```python
from build123d import *

# Parameters (mm, degrees)
BOSS_EXTRUDE2_DEPTH = 5
SKETCH8_R           = 50
CUT_EXTRUDE6_DEPTH  = 20
SKETCH9_OUTSIDE_W   = 10.609
SKETCH9_OUTSIDE_H   = 17.306
SKETCH9_OUTSIDE_R   = 50
CUT_EXTRUDE7_DEPTH  = 20
SKETCH11_W          = 2
SKETCH11_H          = 8
SKETCH11_W_2        = 7
BOSS_EXTRUDE4_DEPTH = 2
CUT_EXTRUDE8_DEPTH  = 18
SKETCH13_R          = 0.3
CUT_EXTRUDE10_DEPTH = 20.940160481
SKETCH14_R          = 0.3
CUT_EXTRUDE11_DEPTH = 20
FILLET1_R           = 0.57
SKETCH15_R          = 16.5
CUT_EXTRUDE12_DEPTH = 20.940160481
SKETCH16_W          = 3.5
SKETCH16_H          = 4.171301815
SKETCH16_H_2        = 4.584730653
CUT_EXTRUDE14_DEPTH = 3.5


# Read off the part's stored shape, not the designer's step: Cut-Extrude8
with BuildPart() as part:
    # Sketch1 → Boss-Extrude2 (new body)
    with BuildSketch(Plane.XY):
        Polygon((0, 0), (0, 8), (2, 8), (2, 5), (5.5, 6), (5.5, 8), (12.5, 8), (12.5, 6), (16, 5), (16, 8), (18, 8), (18, 0), (16, 0), (16, -3), (12.5, -2), (12.5, 0), (5.5, 0), (5.5, -2), (2, -3), (2, 0), align=None)
    extrude(amount=BOSS_EXTRUDE2_DEPTH)

    # Sketch8 → Cut-Extrude6 (cut)
    with BuildSketch(Plane(origin=(0, 0, 0), x_dir=(0, 0, -1), z_dir=(1, 0, 0))):
        with Locations((49, 2.5)):
            Circle(SKETCH8_R)
    extrude(amount=CUT_EXTRUDE6_DEPTH, mode=Mode.SUBTRACT)

    # Sketch9 outside → Cut-Extrude7 (cut)
    with BuildSketch(Plane(origin=(0, 0, 0), x_dir=(0, 0, -1), z_dir=(1, 0, 0))):
        with Locations((-2.8485, 2.5)):
            Rectangle(SKETCH9_OUTSIDE_W, SKETCH9_OUTSIDE_H)
        with Locations((47.1, 2.5)):
            Circle(SKETCH9_OUTSIDE_R, mode=Mode.SUBTRACT)
    extrude(amount=CUT_EXTRUDE7_DEPTH, mode=Mode.SUBTRACT)

    # Sketch11 → Boss-Extrude4 (add)
    with BuildSketch(Plane.XY.offset(4)):
        with Locations((1, 4)):
            Rectangle(SKETCH11_W, SKETCH11_H)
        with Locations((9, 4)):
            Rectangle(SKETCH11_W_2, SKETCH11_H)
        with Locations((17, 4)):
            Rectangle(SKETCH11_W, SKETCH11_H)
    extrude(amount=-BOSS_EXTRUDE4_DEPTH)

    # Cut-Extrude8 outline → Cut-Extrude8 (cut)
    with BuildSketch(Plane(origin=(0, 0, 0), x_dir=(0, 0, -1), z_dir=(1, 0, 0))):
        with BuildLine():
            Line((-4, 0), (-3.037460889, 0))
            ThreePointArc((-3.037460889, 0), (-3.07734981, 4.004827558), (-2.796579359, 8))
            Line((-2.796579359, 8), (-4, 8))
            Line((-4, 8), (-4, 0))
        make_face()
    extrude(amount=CUT_EXTRUDE8_DEPTH, mode=Mode.SUBTRACT)

    # Sketch13 → Cut-Extrude10 (cut, through all)
    with BuildSketch(Plane(origin=(0, 0, 0), x_dir=(0, 0, -1), z_dir=(1, 0, 0))):
        with Locations(Location((-1.799307082, 7.02, 0), (0, 0, 270))):
            Circle(SKETCH13_R)
    extrude(amount=CUT_EXTRUDE10_DEPTH, mode=Mode.SUBTRACT)

    # Sketch14 → Cut-Extrude11 (cut)
    with BuildSketch(Plane(origin=(0, 0, 0), x_dir=(0, 0, -1), z_dir=(1, 0, 0))):
        with Locations(Location((-1.865607241, -1.2, 0), (0, 0, 270))):
            Circle(SKETCH14_R)
    extrude(amount=CUT_EXTRUDE11_DEPTH, mode=Mode.SUBTRACT)

    # Fillet1
    # the kernel refuses this fillet: 0.57 mm, written as the material it takes off along each edge
    with BuildSketch(Plane(origin=(16, 0, 3.037460889), x_dir=(0, 0, -1), z_dir=(1, 0, 0))) as fillet1_piece_1:
        with BuildLine():
            CenterArc((0.545153795, 0.57), FILLET1_R, 182.237689069, 87.762310931)
            ThreePointArc((-0.02441155, 0.547744285), (-0.012956585, 0.273838681), (0, 0))
            Line((0, 0), (0.545153795, 0))
        make_face()
    extrude(amount=3.370719987, mode=Mode.SUBTRACT)
    with BuildSketch(Plane(origin=(14.71001217, 8, 2.796579359), x_dir=(0, 0, -1), z_dir=(1, 0, 0)), Plane(origin=(-1.28998783, 8, 2.796579359), x_dir=(0, 0, -1), z_dir=(1, 0, 0))) as fillet1_piece_2:
        with BuildLine():
            CenterArc((0.513045529, -0.57), FILLET1_R, 90, 84.275973917)
            ThreePointArc((-0.054112356, -0.513149909), (-0.02771814, -0.25650515), (0, 0))
            Line((0, 0), (0.513045529, 0))
        make_face()
    extrude(amount=4.57997566, mode=Mode.SUBTRACT)
    with BuildSketch(Plane(origin=(5.5, 0, 3.037460889), x_dir=(0, 0, -1), z_dir=(1, 0, 0))) as fillet1_piece_3:
        with BuildLine():
            CenterArc((0.545153795, 0.57), FILLET1_R, 182.237689069, 87.762310931)
            ThreePointArc((-0.02441155, 0.547744285), (-0.012956585, 0.273838681), (0, 0))
            Line((0, 0), (0.545153795, 0))
        make_face()
    extrude(amount=7, mode=Mode.SUBTRACT)
    with BuildSketch(Plane(origin=(4.21001217, 8, 2.796579359), x_dir=(0, 0, -1), z_dir=(1, 0, 0))) as fillet1_piece_4:
        with BuildLine():
            CenterArc((0.513045529, -0.57), FILLET1_R, 90, 84.275973917)
            ThreePointArc((-0.054112356, -0.513149909), (-0.02771814, -0.25650515), (0, 0))
            Line((0, 0), (0.513045529, 0))
        make_face()
    extrude(amount=9.57997566, mode=Mode.SUBTRACT)
    with BuildSketch(Plane(origin=(-1.370719987, 0, 3.037460889), x_dir=(0, 0.9990083494743675, 0.044523226303807895), z_dir=(1, 0, 0))) as fillet1_piece_5:
        with BuildLine():
            CenterArc((0.545162753, -0.569991432), FILLET1_R, 89.685852545, 87.762310931)
            Line((-0.024272006, -0.544613193), (0, 0))
            ThreePointArc((0, 0), (0.274143997, 0.000751555), (0.548287995, 0))
        make_face()
    extrude(amount=3.370719987, mode=Mode.SUBTRACT)
    with BuildSketch(Plane(origin=(2, 0, 0.937460889), x_dir=(0, 0.9990278617443559, 0.04408323330360469), z_dir=(-1, 0, 0)), Plane(origin=(19.489241357, 0, 0.937460889), x_dir=(0, 0.9990278617443559, 0.04408323330360409), z_dir=(-1, 0, 0))) as fillet1_piece_6:
        with BuildLine():
            CenterArc((0.595706111, -0.569990001), FILLET1_R, 90.339381978, 92.187220026)
            Line((0.02626023, -0.595117444), (0, 0))
            ThreePointArc((0, 0), (0.296164915, -0.000877144), (0.592329831, 0))
        make_face()
    extrude(amount=3.489241357, mode=Mode.SUBTRACT)
    with BuildSketch(Plane(origin=(3.581343655, 8, 0.696579359), x_dir=(0, 0, 1), z_dir=(-1, 0, 0))) as fillet1_piece_7:
        with BuildLine():
            CenterArc((0.632537462, -0.57), FILLET1_R, 90, 95.594572842)
            ThreePointArc((0.065252578, -0.625568519), (0.033609947, -0.312681655), (0, 0))
            Line((0, 0), (0.632537462, 0))
        make_face()
    extrude(amount=5.16268731, mode=Mode.SUBTRACT)
    with BuildSketch(Plane(origin=(14.081343655, 8, 0.696579359), x_dir=(0, -0.9946037861150897, 0.1037463669027923), z_dir=(-1, 0, 0))) as fillet1_piece_8:
        with BuildLine():
            CenterArc((0.632547622, 0.569988725), FILLET1_R, 174.045055794, 95.594572842)
            Line((0.065623464, 0.629124155), (0, 0))
            ThreePointArc((0, 0), (0.314481268, 0.000988994), (0.628962535, 0))
        make_face()
    extrude(amount=10.16268731, mode=Mode.SUBTRACT)
    with BuildSketch(Plane(origin=(19.581343655, 8, 0.696579359), x_dir=(0, -0.9946037861150897, 0.1037463669027923), z_dir=(-1, 0, 0))) as fillet1_piece_9:
        with BuildLine():
            CenterArc((0.632547622, 0.569988725), FILLET1_R, 174.045055794, 95.594572842)
            Line((0.065623464, 0.629124155), (0, 0))
            ThreePointArc((0, 0), (0.314481268, 0.000988994), (0.628962535, 0))
        make_face()
    extrude(amount=5.16268731, mode=Mode.SUBTRACT)
    with BuildSketch(Plane(origin=(12.5, 0, 0.937460889), x_dir=(0, 0.9990278617443559, 0.04408323330360469), z_dir=(-1, 0, 0))) as fillet1_piece_10:
        with BuildLine():
            CenterArc((0.595706111, -0.569990001), FILLET1_R, 90.339381978, 92.187220026)
            Line((0.02626023, -0.595117444), (0, 0))
            ThreePointArc((0, 0), (0.296164915, -0.000877144), (0.592329831, 0))
        make_face()
    extrude(amount=7, mode=Mode.SUBTRACT)

    # Sketch15 → Cut-Extrude12 (cut, through all)
    with BuildSketch(Plane.XY):
        with Locations((9, -11.34889303)):
            Circle(SKETCH15_R)
    extrude(amount=CUT_EXTRUDE12_DEPTH, mode=Mode.SUBTRACT)

    # Sketch16 → Cut-Extrude14 (cut)
    with BuildSketch(Plane.XY.offset(5.6)):
        with Locations((3.75, 4.184345942)):
            Rectangle(SKETCH16_W, SKETCH16_H)
        with Locations((14.25, 4.391060361)):
            Rectangle(SKETCH16_W, SKETCH16_H_2)
    extrude(amount=-CUT_EXTRUDE14_DEPTH, mode=Mode.SUBTRACT)


solid = part.part
```
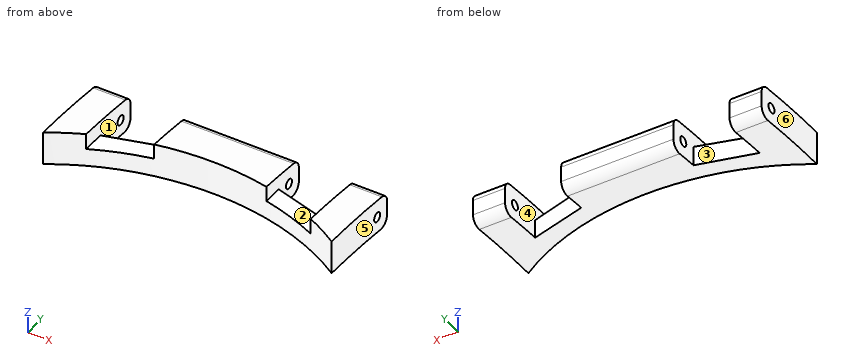
Could you check a few things on this model? Use its own coordinates, in mm. Face numbers are marked on the shaded views. A direction names the side the tool comes from. Give positions to 0.01 mm unless a question says otherwise; leave off trailing zeros. Write each loop counter-clockwise with the first axis right and the second up, starting at its lowest first coordinate (ties: lowest second). Pieces come first, ordered by that corner, then holes. Notation, with made-up numbers: (-31.5, -11) -> (-8.5, -11) arc R8 ccw to (-8.5, -5) -> close; hole circle Ø5 at (-8.75, 25). An arc over 180 degrees is marked (long way). Write each question's results on one line, items separated by ' | '.
1. I need wall thicknesses on L1, parallel to X at y = 6.2, z = 0.95; L2, parallel to X at y = 4.3, z = 2.3; L3, parallel to Z at x = 16.7, y = 7.02. Which ranges of each line are inside material? Lowest first, please.
Check sheet entries:
L1: x = 0 to 2, 5.5 to 12.5, 16 to 18 | L2: x = 0 to 2, 16 to 18 | L3: z = 0.8 to 1.5, 2.1 to 2.9
2. On a 3-axis mill with a long thin cutter (end or side, diameter ignored), from which of +Z, -Z, +X, -X, +Y, -Y can I reach the whole of each face in a straight line? I mean the marked faces 1, 2 and 3. Say none if no direction works.
Check sheet entries:
face 1: +Z, +Y | face 2: +Z, +Y, -Y | face 3: +Z, -Z, +Y
3. I want a section at D-D, the plane x = 7.5. Write out the boundary of the cut face in (y, z).
Check sheet entries:
outline: (5.08, 0.93) arc R50 cw to (7.37, 0.76) arc R0.57 ccw to (8, 1.33) -> (8, 2.28) arc R0.57 ccw to (7.49, 2.85) arc R50 ccw to (5.08, 3.03) -> close; hole circle Ø0.6 at (7.02, 1.8)
4. If we mould it in two halves opening along X, with no side actions, what happens to the marked faces 4, 5 and 6? For each: released by +X, released by -X, zero draft, split by the parting line, or undercut.
Check sheet entries:
face 4: undercut | face 5: released by +X | face 6: released by -X
5. I want a section at A-A, the plane z = 2.5. Write out the boundary of the cut face in (x, y).
Check sheet entries:
outline: (0, 2.48) arc R16.5 cw to (2, 3.59) -> (2, 7.96) -> (0, 7.96) -> close; (5.5, 4.78) arc R16.5 cw to (12.5, 4.78) -> (12.5, 7.96) -> (5.5, 7.96) -> close; (16, 3.59) arc R16.5 cw to (18, 2.48) -> (18, 7.96) -> (16, 7.96) -> close
6. I want a section at C-C, the plane y = 2.95. Write out the boundary of the cut face in (x, z).
Check sheet entries:
outline: (0, 1) -> (0.77, 1) -> (0.77, 3.1) -> (0, 3.1) -> close; (17.23, 1) -> (18, 1) -> (18, 3.1) -> (17.23, 3.1) -> close
7. I want a section at B-B, the plane y = 7.02. Write out the boundary of the cut face in (x, z), then the cut area to 3 significant figures.
Check sheet entries:
outline: (0, 0.8) -> (2, 0.8) -> (2, 1.5) -> (0, 1.5) -> close; (0, 2.1) -> (2, 2.1) -> (2, 2.9) -> (0, 2.9) -> close; (5.5, 0.8) -> (12.5, 0.8) -> (12.5, 1.5) -> (5.5, 1.5) -> close; (5.5, 2.1) -> (12.5, 2.1) -> (12.5, 2.9) -> (5.5, 2.9) -> close; (16, 0.8) -> (18, 0.8) -> (18, 1.5) -> (16, 1.5) -> close; (16, 2.1) -> (18, 2.1) -> (18, 2.9) -> (16, 2.9) -> close | area: 16.5 mm²
8. Will these pins go through, and if not, where does the flat tip stop? pin 1 Ø2 at (x, y) = (14.5, 5) entering from +Z; pin 2 Ø3 at (x, y) = (14, 4) entering from -Z.
Check sheet entries:
pin 1: stops at z = 2.1 | pin 2: stops at z = 0.91
